Autodesk Inventor part; units mm, degrees
ref_plane "YZ Plane" through (0, 0, 0) normal (1, 0, 0) x (0, 1, 0)
ref_plane "XZ Plane" through (0, 0, 0) normal (0, 1, 0) x (-1, 0, 0)
ref_plane "XY Plane" through (0, 0, 0) normal (0, 0, 1) x (1, 0, 0)
sketch "Skizze1" plane through (0, 0, 0) normal (0, 0, 1) x (1, 0, 0)
  line L0 (-14.1284, 0) -> (-14.1284, 11)
  line L1 (-14.1284, 11) -> (-12.5284, 11)
  line L2 (-12.5284, 11) -> (-12.5284, 1.6)
  line L3 (-12.5284, 1.6) -> (6.7716, 1.6)
  line L4 (6.7716, 1.6) -> (6.7716, 11)
  line L5 (6.7716, 11) -> (8.3716, 11)
  line L6 (8.3716, 11) -> (8.3716, 0)
  line L7 (8.3716, 0) -> (-14.1284, 0)
  line L8 (-16.6284, 14) -> (10.8716, 14)
  line L9 (10.8716, 14) -> (10.8716, -3)
  line L10 (10.8716, -3) -> (-16.6284, -3)
  line L11 (-16.6284, -3) -> (-16.6284, 14)
  line L12 (-12.5284, 9.5) -> (6.7716, 9.5)
  point P0 (0, 0)
  dimension "d0" = 11
  dimension "d1" = 1.6
  dimension "d2" = 19.3
  dimension "d3" = 1.6
  dimension "d4" = 1.6
  dimension "d5" = 3
  dimension "d6" = 3
  dimension "d7" = 2.5
  dimension "d8" = 2.5
  dimension "d9" = 1.5
extrude "Extrusion1" add sketch "Skizze1" along normal blind 30
fillet "Rundung1" radius 2 12 edges at (10.8716, 14, 15) (10.8716, -3, 15) (-16.6284, -3, 15) (-16.6284, 14, 15) (-2.8784, 14, 30) (-16.6284, 5.5, 30) (-2.8784, -3, 30) (10.8716, 5.5, 30) (10.8716, 5.5, 0) (-2.8784, -3, 0) (-2.8784, 14, 0) (-16.6284, 5.5, 0)
sketch "Skizze2" plane through (10.8716, -1, 28) normal (1, 0, 0) x (0, 0, -1)
  line L0 (0, 15) -> (26, 15)
  line L1 (8, 15) -> (4.25, 22)
  line L2 (4.25, 22) -> (21.75, 22)
  line L3 (21.75, 22) -> (18, 15)
  line L4 (28, 0) -> (28, 13)
  point P0 (28, 1)
  dimension "d13" = 10
  dimension "d15" = 7
  dimension "d16" = 3.75
  dimension "d17" = 3.75
  dimension "d18" = 17.5
  dimension "d19" = 10
extrude "Extrusion2" add sketch "Skizze2" against normal blind 27.5
sketch "Skizze4" plane through (10.8716, 21, 23.75) normal (0, 1, 0) x (1, 0, 0)
  line L0 (-25.5, 21.75) -> (-25.5, -4.25)
  line L1 (-27.5, 3.75) -> (-27.5, 0)
  line L2 (-25.5, 17.5243) -> (-27.5, 17.5243)
  line L3 (-27.5, 17.5243) -> (-27.5, 0)
  line L4 (-27.5, 0) -> (-25.5, 0)
  line L5 (-25.5, 0) -> (-25.5, 17.5243)
  line L6 (0, 17.5) -> (-27.5, 17.5)
  line L7 (-2, 3.75) -> (-2, -4.25)
  line L8 (0, 17.5) -> (-2, 17.5)
  line L9 (-2, 17.5) -> (-2, 0)
  line L10 (-2, 0) -> (0, 0)
  line L11 (0, 0) -> (0, 17.5)
  point P0 (-10.8716, 23.75)
extrude "Extrusion4" cut sketch "Skizze4" against normal blind 7
properties part number "Schienenläufermitkeil_22.5"
Input: part model. Units: mm. Frame: model coordinates. A direction names the side the tool comes from. Coordinates: 2 decimals unless noted, no trailing zeros. Write each loop counter-clockwise with the first axis right and the second up, starting at its lowest first coordinate (ties: lowest second). Pieces come first, ordered by that corner, then holes. Notation, with made-up numbers: M 25,38 L 39,38 A32 cw 39,65 Z; hole C 53,73.25 d11. An arc over 180 degrees is marked long. Use one line per item in the form item = value.
Q1. Section A-A (z = 21.5). Return loops of the section in (x, y).
Answer below:
outline = M -16.63,-1 A2 ccw -14.63,-3 L 8.87,-3 A2 ccw 10.87,-1 L 10.87,12 A2 ccw 8.87,14 L -14.63,14 A2 ccw -16.63,12 Z; M -14.63,16.8 L 8.87,16.8 L 8.87,21 L -14.63,21 Z; hole M -14.13,0 L 8.37,0 L 8.37,11 L 6.77,11 L 6.77,9.5 L -12.53,9.5 L -12.53,11 L -14.13,11 Z
Q2. Set-up query: faces 1 (the face through (8.872, 18, 15)), 2 (the face through (-3, 14, 24)), 3 (the face through (8, 11, 15)). Return all of +Z, -Z, +X, -X, +Y, -Y with unobstructed straight access to the full face (end or side cutting, diameter ignored); none if empty.
Answer below:
face_1 = +Z, -Z, +X, +Y
face_2 = +Z, +X, -X
face_3 = +Z, -Z
Q3. First-contact query: pin 1 (1 mm diameter, centred on x = -13.5, y = 17, fed in from -Z) (3 decimals); pin 2 (5.5 mm diameter, centred on y = 16.5, z = 18.5, fed in from -X); pin 3 (5.5 mm diameter, centred on y = 19, z = 18.5, fed in from +X). Flat tips, straight axial feed; report the tip coordinate or a pass-through.
Answer below:
pin_1 = 8.125
pin_2 = -15.6
pin_3 = 8.87
Q4. Material intervals for probe 1 along X at (y, z) = (10.75, 4); probe 2 along Y at (x, z) = (-6, 10.5); probe 3 along X at (y, z) = (1.25, 12), sorted ascending. Write a range as from..to.
Answer below:
probe_1 = -16.63..-14.13, -12.53..6.77, 8.37..10.87
probe_2 = -3..0, 9.5..21
probe_3 = -16.63..-14.13, 8.37..10.87
Q5. Section D-D (z = 12). Return loops of the section in (x, y).
Answer below:
outline = M -16.63,-1 A2 ccw -14.63,-3 L 8.87,-3 A2 ccw 10.87,-1 L 10.87,12 A2 ccw 8.87,14 L 8.87,21 L -14.63,21 L -14.63,14 A2 ccw -16.63,12 Z; hole M -14.13,0 L 8.37,0 L 8.37,11 L 6.77,11 L 6.77,9.5 L -12.53,9.5 L -12.53,11 L -14.13,11 Z
Q6. Section C-C (y = 3). Return loops of the section in (x, z), plus the area to 3 significant figures.
Answer below:
outline = M -16.63,2 A2 ccw -14.63,0 L -14.13,0 L -14.13,30 L -14.63,30 A2 ccw -16.63,28 Z; M 8.37,0 L 8.87,0 A2 ccw 10.87,2 L 10.87,28 A2 ccw 8.87,30 L 8.37,30 Z
area = 147 mm²
Q7. Section B-B (x = -6). Return loops of the section in (y, z).
Answer below:
outline = M -3,2 A2 ccw -1,0 L 0,0 L 0,30 L -1,30 A2 ccw -3,28 Z; M 9.5,0 L 12,0 A2 ccw 14,2 L 14,10 L 21,6.25 L 21,23.75 L 14,20 L 14,28 A2 ccw 12,30 L 9.5,30 Z
Q8. Draft query along Y for faces 4 (the face through (-14.128, 5, 15)), 5 (the face through (-2, 10, 0)), 6 (the face through (-3, 21, 15)). Return one class per face: released by +Y, released by -Y, zero draft, split by the parting line, or undercut.
Answer below:
face_4 = undercut
face_5 = zero draft
face_6 = released by +Y
